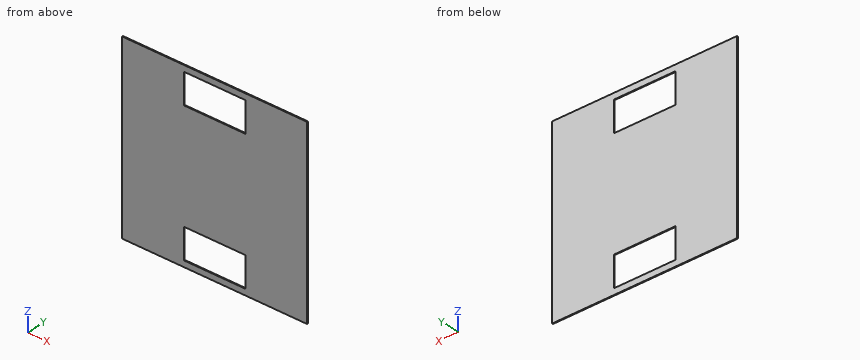
Autodesk Inventor part; units mm, degrees
ref_plane "YZ Plane" through (0, 0, 0) normal (1, 0, 0) x (0, 1, 0)
ref_plane "XZ Plane" through (0, 0, 0) normal (0, 1, 0) x (-1, 0, 0)
ref_plane "XY Plane" through (0, 0, 0) normal (0, 0, 1) x (1, 0, 0)
sketch "Boceto1" plane through (0, 0, 0) normal (0, 1, 0) x (-1, 0, 0)
  line L0 (16.7386, 18.54) -> (16.7386, -281.46)
  line L1 (16.7386, -281.46) -> (316.7386, -281.46)
  line L2 (316.7386, -281.46) -> (316.7386, 18.54)
  line L3 (316.7386, 18.54) -> (16.7386, 18.54)
  point P0 (0, 0)
  dimension "d2" = 300
  dimension "d3" = 300
extrude "Extrusión1" add sketch "Boceto1" along normal mid plane 1.5
sketch "Boceto2" plane through (0, 0.75, 0) normal (0, 1, 0) x (1, 0, 0)
  line L0 (-316.7386, -18.54) -> (-16.7386, -18.54)
  line L1 (-16.7386, 281.46) -> (-316.7386, 281.46)
  line L2 (-316.7386, 281.46) -> (-316.7386, -18.54)
  line L3 (-316.7386, 131.46) -> (-16.7386, 131.46)
  line L4 (-16.7386, -18.54) -> (-16.7386, 281.46)
  line L5 (-166.7386, -18.54) -> (-166.7386, -8.54)
  line L6 (-166.7386, 281.46) -> (-166.7386, 271.46)
  line L7 (-166.7386, 271.46) -> (-116.7386, 271.46)
  line L8 (-116.7386, 271.46) -> (-116.7386, 221.46)
  line L9 (-116.7386, 221.46) -> (-166.7386, 221.46)
  line L10 (-166.7386, 221.46) -> (-216.7386, 221.46)
  line L11 (-216.7386, 221.46) -> (-216.7386, 271.46)
  line L12 (-216.7386, 271.46) -> (-166.7386, 271.46)
  line L13 (-166.7386, -8.54) -> (-216.7386, -8.54)
  line L14 (-216.7386, -8.54) -> (-216.7386, 41.46)
  line L15 (-216.7386, 41.46) -> (-166.7386, 41.46)
  line L16 (-116.7386, 41.46) -> (-166.7386, 41.46)
  line L17 (-116.7386, -8.54) -> (-166.7386, -8.54)
  line L18 (-116.7386, 41.46) -> (-116.7386, -8.54)
  line L19 (-166.7386, -18.54) -> (-166.7386, -8.54)
  line L20 (-166.7386, 271.46) -> (-166.7386, 281.46)
  point P0 (0, 0)
  dimension "d6" = 10
  dimension "d7" = 10
  dimension "d8" = 50
  dimension "d9" = 50
  dimension "d10" = 50
  dimension "d11" = 50
  dimension "d12" = 50
extrude "Extrusión2" cut sketch "Boceto2" against normal blind 4 contours L13 L14 L15 L16 L18 L17 | L7 L8 L9 L10 L11 L12
properties part number "base 30x30"
Geometry check sheet. Reference: the model listing, model coordinates, mm. Round coordinates to 2 decimals unless told otherwise and drop trailing zeros. Write each loop counter-clockwise with the first axis right and the second up, starting at its lowest first coordinate (ties: lowest second). Pieces come first, ordered by that corner, then holes. Notation, with made-up numbers: (75, 71.25) -> (111, 71.25) arc R37 cw to (111, 109.25) -> close; hole circle Ø7 at (57, 6). An arc over 180 degrees is marked (long way). Put each result on its own line as item: value.
1) Cross-section at C-C, the plane y = 0.4. Enter the section's corners in (x, z), plus the area to 3 significant figures.
Recorded:
outline: (-316.74, -281.46) -> (-16.74, -281.46) -> (-16.74, 18.54) -> (-316.74, 18.54) -> close; hole (-216.74, -271.46) -> (-116.74, -271.46) -> (-116.74, -221.46) -> (-216.74, -221.46) -> close; hole (-216.74, -41.46) -> (-116.74, -41.46) -> (-116.74, 8.54) -> (-216.74, 8.54) -> close
area: 80,000 mm2
2) Thickness scan on probe 1 along Z at (x, y) = (-167, -0.05); probe 2 along X at (y, z) = (0.4, -20.5). Record the ranges inside material, lowest first. Write a range as from..to.
Recorded:
probe 1: z = -281.46..-271.46, -221.46..-41.46, 8.54..18.54
probe 2: x = -316.74..-216.74, -116.74..-16.74
3) Cross-section at A-A, the plane z = -28.5. Enter the section's corners in (x, y), plus the area to 3 significant figures.
Recorded:
outline: (-316.74, -0.75) -> (-216.74, -0.75) -> (-216.74, 0.75) -> (-316.74, 0.75) -> close; (-116.74, -0.75) -> (-16.74, -0.75) -> (-16.74, 0.75) -> (-116.74, 0.75) -> close
area: 300 mm2
4) Cross-section at B-B, the plane x = -134. Enter the section's corners in (y, z), plus the area to 3 significant figures.
Recorded:
outline: (-0.75, -281.46) -> (0.75, -281.46) -> (0.75, -271.46) -> (-0.75, -271.46) -> close; (-0.75, -221.46) -> (0.75, -221.46) -> (0.75, -41.46) -> (-0.75, -41.46) -> close; (-0.75, 8.54) -> (0.75, 8.54) -> (0.75, 18.54) -> (-0.75, 18.54) -> close
area: 300 mm2
